Study the drawing (mm; zero at the part's minimum x, y, z) and answer. Give positions to 0.01 mm unless a question says otherwise; leave off trailing zeros. Order: outer loops, then holes, each group sorted by start corner. A loop starts at its lowest first (then second) coordinate and runs counter-clockwise, first axis right, second up.
Item 1: A cutting plane is placed at A-A (y = 3.75). Write down the section's boundary in (x, z), plus the area to 3 significant figures.
Item 2: A cutting plane is placed at C-C (x = 63). Write down the section's boundary in (y, z), plus the area to 3 significant figures.
Item 3: Find the intervals of material crossed by line 1 along X through (y, z) = (8.5, 139); line 2 along Z through (x, y) = (62, 16.75); line 3 along Z through (x, y) = (77, 14), in increasing order.
Item 4: A cutting plane is placed at B-B (z = 61.5). Write down the section's boundary in (x, y).
Item 5: Given pin 1 Ø3 at (y, z) = (2.5, 69) entering from +X; pin 2 Ø8 at (y, z) = (2, 48) entering from +X, each flat-ended and moving along its own axis, determine where each tip first touches the part or whether it passes through.
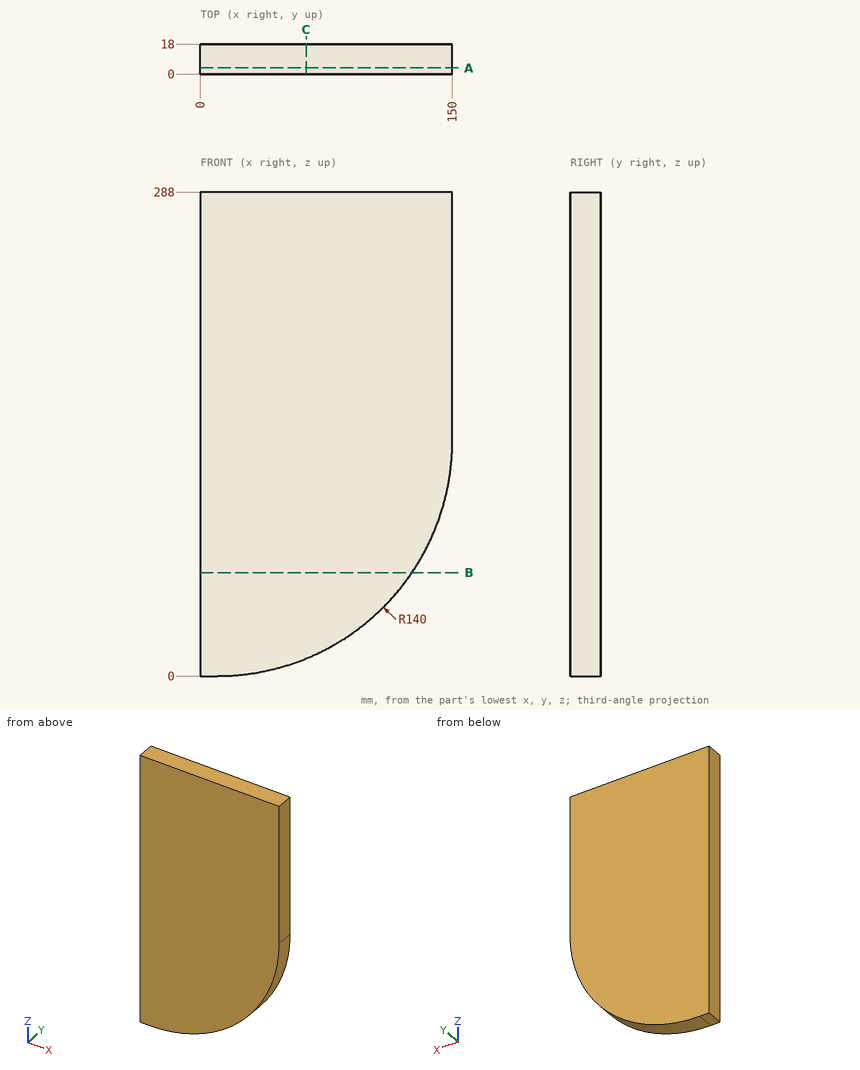
Response values:
1. outline: (0, 0) - (10, 0) arc R140 ccw to (150, 140) - (150, 288) - (0, 288) - close
1. area: 39,000 mm2
2. outline: (0, 10.42) - (18, 10.42) - (18, 288) - (0, 288) - close
2. area: 5,000 mm2
3. line 1: x = 0 to 150
3. line 2: z = 10.02 to 288
3. line 3: z = 17.07 to 288
4. outline: (0, 0) - (125.92, 0) - (125.92, 18) - (0, 18) - close
5. pin 1: stops at x = 131.53
5. pin 2: stops at x = 118.89
